```python
from build123d import *

# Parameters (mm, degrees)
SKETCH1_R           = 21
SKETCH1_R_2         = 4
BOSS_EXTRUDE1_DEPTH = 48
SKETCH2_R           = 19
CUT_EXTRUDE1_DEPTH  = 42
SKETCH3_R           = 6
SKETCH3_R_2         = 4
BOSS_EXTRUDE2_DEPTH = 20
SKETCH7_R           = 5
SKETCH7_R_2         = 4


with BuildPart() as part:
    # Sketch1 → Boss-Extrude1 (new body)
    with BuildSketch(Plane(origin=(0, 0, 0), x_dir=(1, 0, 0), z_dir=(0, 1, 0))):
        Circle(SKETCH1_R)
        with Locations((0, -10.495775772)):
            Circle(SKETCH1_R_2, mode=Mode.SUBTRACT)
        with Locations((0, 8.217839423)):
            Circle(SKETCH1_R_2, mode=Mode.SUBTRACT)
    extrude(amount=BOSS_EXTRUDE1_DEPTH)

    # Sketch2 → Cut-Extrude1 (cut)
    with BuildSketch(Plane.XZ):
        Circle(SKETCH2_R)
    extrude(amount=-CUT_EXTRUDE1_DEPTH, mode=Mode.SUBTRACT)

    # Sketch3 → Boss-Extrude2 (add)
    with BuildSketch(Plane(origin=(0, 48, 0), x_dir=(1, 0, 0), z_dir=(0, 1, 0))):
        with Locations((0, 8.217839423)):
            Circle(SKETCH3_R)
        with Locations((0, 8.217839423)):
            Circle(SKETCH3_R_2, mode=Mode.SUBTRACT)
        with Locations((0, -10.495775772)):
            Circle(SKETCH3_R)
        with Locations((0, -10.495775772)):
            Circle(SKETCH3_R_2, mode=Mode.SUBTRACT)
    extrude(amount=BOSS_EXTRUDE2_DEPTH)

    # Sweep9: sweep along a path in Sketch4
    with BuildLine(Plane(origin=(0, 0, 0), x_dir=(0, 0, -1), z_dir=(1, 0, 0))) as sweep9_path:
        Line((8.160870432, 48), (8.160870432, -252))
        ThreePointArc((8.160870432, -252), (-1.16745267, -261.328323102), (-10.495775772, -252))
        Line((-10.495775772, -252), (-10.495775772, 48))
    # Sketch7 → Sweep9 (sweep)
    with BuildSketch(Plane.XZ.offset(-42)):
        with Locations((0, 10.495775772)):
            Circle(SKETCH7_R)
        with Locations((0, 10.495775772)):
            Circle(SKETCH7_R_2, mode=Mode.SUBTRACT)
    sweep(path=sweep9_path.line)


solid = part.part
```
Source: CAD feature listing. Evaluate the final solid. Frame: model axes, mm. A direction names the side the tool comes from. Coordinates: 2 decimals unless noted, no trailing zeros. Loops run counter-clockwise (first coordinate to the right, second up) from the corner with the lowest first, then second, coordinate; pieces in that order, holes last. Notation, with made-up numbers: M -34.5,-15 L -13.5,-15 A29 ccw -13.5,10 Z; hole C -28,49 d4. An arc over 180 degrees is marked long. Use CSV: the item, a comma, the result in double quotes.
(1) Line query: line 1 (Z direction, x = 0, y = 55.75); line 2 (Z direction, x = 0, y = -190); line 3 (Z direction, x = 0, y = 27.5). Output: solid intervals per line, ascending. Write a range as [from, to].
Answers follow:
line 1,"[-14.22, -12.22], [-4.22, -2.22], [4.5, 6.5], [14.5, 16.5]"
line 2,"[-13.16, -12.16], [-4.16, -3.16], [5.5, 6.5], [14.5, 15.5]"
line 3,"[-21, -19], [-13.16, -12.16], [-4.16, -3.16], [5.5, 6.5], [14.5, 15.5], [19, 21]"
(2) Contact query for flat-ended pins moving along their axis: pin 1 (12 mm diameter, centred on x = -14, z = -1, fed in from +Y); pin 2 (10 mm diameter, centred on x = -7.5, y = -12.5, fed in from +Z); pin 3 (4.5 mm diameter, centred on x = -0.5, z = -6.5, fed in from -Y). Output: stop coordinate, or through.
Answers follow:
pin 1,"y = 48"
pin 2,"z = 14.83"
pin 3,"y = -265.25"
(3) Cut plane B-B on x = 0. Give the number of separate pieces and of enclosed holes in the cut face, and give its area (3 significant figures).
Answers follow:
separate pieces,"2"
enclosed holes,"1"
area,"1,720 mm²"
(4) Draft query along X for faces 1 (the face through (8.767, 20.706, -16.856)), 2 (the face through (20.03, 23.66, -6.31)), 3 (the face through (4, 68, -7)). Return one class per face: pulls with the +X half, pulls with the -X half, needs draft (parallel to the pull), parting line crosses it, or undercut.
Answers follow:
face 1,"undercut"
face 2,"parting line crosses it"
face 3,"needs draft"
(5) Cut plane A-A on y = 30.5. Return loops of the section in (x, z).
Answers follow:
outline,"C 0,0 d42; C 0,-8.16 d10; C 0,10.5 d10; hole C 0,0 d38; hole C 0,-8.16 d8; hole C 0,10.5 d8"
(6) Cut plane C-C on y = -104. Return loops of the section in (x, z).
Answers follow:
outline,"C 0,-8.16 d10; C 0,10.5 d10; hole C 0,-8.16 d8; hole C 0,10.5 d8"
(7) Reachability of faces 4 (the face through (4, 68, 12)), 5 (the face through (-1.301, 57.86, 16.353)), 6 (the face through (2.69, -102.94, 6.28)) from +Z, -Z, +X, -X, +Y, -Y: full face, straight path, thin tool, end or side. Return the list, or none.
Answers follow:
face 4,"+Z, -Z, +X, -X, +Y"
face 5,"+Y"
face 6,"none"
